Answer from the drawing. Dimensions are ordinates in mm from the lowest x, y and z of the part. A direction names the side the tool comes from. Round coordinates to 2 decimals unless told otherwise and drop trailing zeros. Write each loop counter-clockwise with the first axis right and the second up, starting at its lowest first coordinate (ties: lowest second). Pieces come first, ordered by that corner, then holes. Notation, with made-up numbers: (-21, 71.5) - (33, 71.5) arc R8 cw to (33, 79.5) - close; hole circle Ø5 at (18, 33). An arc over 180 degrees is marked (long way). Use a Markdown table: item, result. Add a question column.
1) A cutting plane is placed at A-A (y = 6). Give the vertices of the cut face in (x, z) (3 decimals).
2) A tool of negligible diameter and unlimited length cuts with its end or side. For the marked faces 4 and 5, from which of +Z, -Z, +X, -X, +Y, -Y can it reach the whole face along a straight path? Write none if from no direction.
3) A cutting plane is placed at C-C (z = 3.2). Give the vertices of the cut face in (x, y) (3 decimals), then the cut area to 3 significant figures.
4) A cutting plane is placed at D-D (z = 0.7). Give the vertices of the cut face in (x, y) (3 decimals), then the cut area to 4 significant figures.
5) Determine the mould class of the marked faces 1, 2 and 3 for opening direction X: +X half, -X half, draft (parallel to the pull), parting line (faces both ways), or undercut.
6) Find the intervals of material crossed by probe 1 along Y at (x, z) = (6, 2.35) (3 decimals); probe 2 along Z at (x, y) = (9, 10.5); probe 3 along X at (y, z) = (3.25, 0.8), in increasing order. Write a range as from..to.
7) Each of these flat-tipped pins is pushed along its axis until it touches: P1, Ø5, axis at x = 1, y = 8, coming from the +Z side; P2, Ø1.5, axis at y = 7, z = 1.5, coming from the -X side; P3, Ø2, axis at x = 3, z = 1, coming from the -Y side. Where does it stop, or does it pass through?
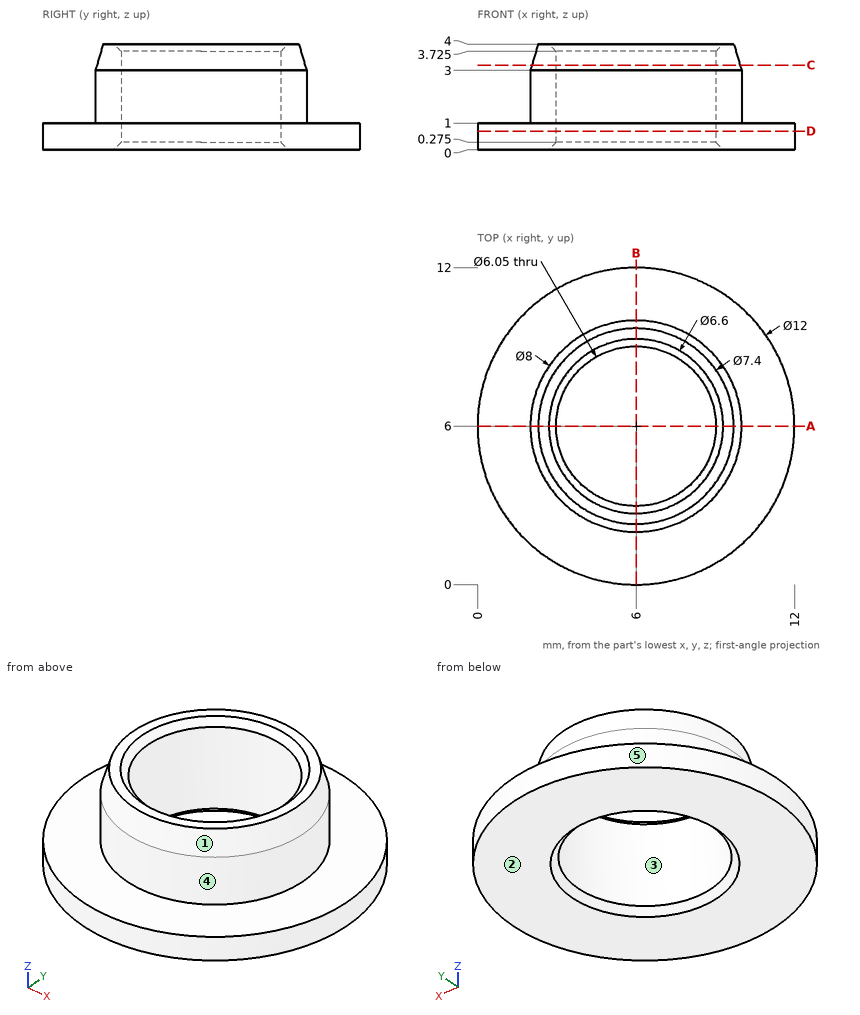
Entries:
| question | item | result |
|---|---|---|
| 1 | outline | (0, 0) - (2.7, 0) - (2.975, 0.275) - (2.975, 3.725) - (2.7, 4) - (2.3, 4) - (2, 3) - (2, 1) - (0, 1) - close; (9.025, 0.275) - (9.3, 0) - (12, 0) - (12, 1) - (10, 1) - (10, 3) - (9.7, 4) - (9.3, 4) - (9.025, 3.725) - close |
| 2 | face 4 | +Z |
| 2 | face 5 | +Z, -Z |
| 3 | outline | circle Ø7.88 at (6, 6); hole circle Ø6.05 at (6, 6) |
| 3 | area | 20.0 mm² |
| 4 | outline | circle Ø12 at (6, 6); hole circle Ø6.05 at (6, 6) |
| 4 | area | 84.35 mm² |
| 5 | face 1 | parting line |
| 5 | face 2 | draft |
| 5 | face 3 | undercut |
| 6 | probe 1 | y = 2..2.975, 9.025..10 |
| 6 | probe 2 | z = 0..1 |
| 6 | probe 3 | x = 0.67..4.74, 7.26..11.33 |
| 7 | P1 | stops at z = 4 |
| 7 | P2 | stops at x = 0.02 |
| 7 | P3 | stops at y = 0.34 |
